```python
from build123d import *

# Parameters (mm, degrees)
ESQUISSE1_R        = 1.75
BOSS_EXTRU_1_DEPTH = 1.5
ESQUISSE2_W        = 96.5
ESQUISSE2_H        = 181
BOSS_EXTRU_2_DEPTH = 41


with BuildPart() as part:
    # Esquisse1 → Boss.-Extru.1 (new body)
    with BuildSketch(Plane.XY):
        with BuildLine():
            ThreePointArc((-8.5, -195.25), (-6.75, -193.5), (-5, -195.25))
            Line((-5, -195.25), (-5, -198))
            Line((-5, -198), (0, -198))
            Line((0, -198), (0, 0))
            Line((0, 0), (-98, 0))
            Line((-98, 0), (-98, -198))
            Line((-98, -198), (-8.5, -198))
            Line((-8.5, -198), (-8.5, -195.25))
        make_face()
        with Locations((-92, -3)):
            Circle(ESQUISSE1_R, mode=Mode.SUBTRACT)
    extrude(amount=BOSS_EXTRU_1_DEPTH)

    # Esquisse2 → Boss.-Extru.2 (add)
    with BuildSketch(Plane.XY.offset(1.5)):
        with Locations((-48.25, -102.5)):
            Rectangle(ESQUISSE2_W, ESQUISSE2_H)
        Polygon((-98, 0), (-98, -198), (-96.5, -198), (-96.5, -193), (-96.5, -12), (-96.5, 0), align=None)
    extrude(amount=BOSS_EXTRU_2_DEPTH)


solid = part.part
```
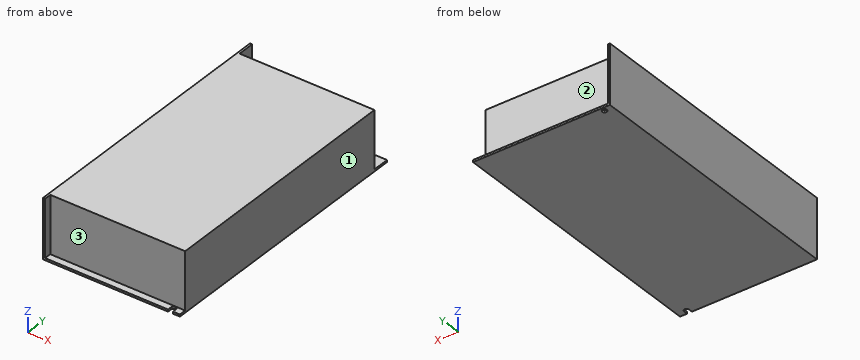
Geometry: final body of the model. Coordinates: model frame, mm. Face numbers are marked on the shaded views. A direction names the side the tool comes from. Coordinates: 2 decimals unless noted, no trailing zeros. Order: outer loops, then holes, each group sorted by start corner. A loop starts at its lowest first (then second) coordinate and runs counter-clockwise, first axis right, second up. Notation, with made-up numbers: (-20.5, 68.5) - (17.5, 68.5) arc R9 ccw to (17.5, 74.5) - close; hole circle Ø9 at (21.5, 41). An arc over 180 degrees is marked (long way). Return JSON: item names as keys, results as strings. Group by question number.
1. Cut plane A-A (z = 14). Output: boundary loops of the cut face in (x, y), plus the area to 3 significant figures.
2. Cut plane B-B (x = -58). Output: boundary loops of the cut face in (y, z), plus the area to 3 significant figures.
3. Pin query (flat end, axial travel): pin 1 (8 mm diameter, centred on x = -48, z = 19.5, fed in from -Y); pin 2 (5 mm diameter, centred on x = -15, z = 24, fed in from +Y); pin 3 (3.5 mm diameter, centred on x = -68, y = -6, fed in from +Z). Return the tip coordinate at first contact, or that it passes through.
4. Set-up query: the marked faces 1, 2 and 3. Return all of +Z, -Z, +X, -X, +Y, -Y with unobstructed straight access to the full face (end or side cutting, diameter ignored); none if empty.
5. Material intervals for line 1 along Y through (x, z) = (-92, 0.7); line 2 along Y through (x, z) = (-25.5, 10.5); line 3 along Z through (x, y) = (-10.5, -11), sorted ascending. Write a range as [from, to].
Resolved:
{
 "1": {"outline": "(-98, -198) - (-96.5, -198) - (-96.5, -193) - (0, -193) - (0, -12) - (-96.5, -12) - (-96.5, 0) - (-98, 0) - close", "area": "17,800 mm²"},
 "2": {"outline": "(-198, 0) - (0, 0) - (0, 1.5) - (-12, 1.5) - (-12, 42.5) - (-193, 42.5) - (-193, 1.5) - (-198, 1.5) - close", "area": "7,720 mm²"},
 "3": {"pin 1": "stops at y = -193", "pin 2": "stops at y = -12", "pin 3": "stops at z = 1.5"},
 "4": {"face 1": "+Z, -Z, +X, +Y, -Y", "face 2": "+Z, +X, +Y", "face 3": "+Z, +X, -Y"},
 "5": {"line 1": "y = [-198, -4.75], [-1.25, 0]", "line 2": "y = [-193, -12]", "line 3": "z = [0, 1.5]"}
}
